Could you check a few things on this model? Use its own coordinates, in mm. Face numbers are marked on the shaded views. A direction names the side the tool comes from. Coordinates: 2 decimals unless noted, no trailing zeros. Order: outer loops, then holes, each group sorted by start corner. A loop starts at its lowest first (then second) coordinate and runs counter-clockwise, first axis right, second up. Notation, with made-up numbers: (-2, -22.5) - (3, -22.5) arc R16 cw to (3, 5.5) - close; hole circle Ø6 at (-19.5, 51.5). An arc over 180 degrees is marked (long way). Answer as a JSON object with one key per item and string values. Group by question number.
(1) Imagine slicing it at D-D, the plane y = 109.5. Write out the boundary of the cut face in (x, z), and give its area (3 significant figures).
(2) Imagine slicing it at A-A, the plane z = -72. Write out the boundary of the cut face in (x, y), and give its area (3 significant figures).
(3) Please list where these lines run through material, in increasing order: probe 1 along Y at (x, z) = (-10, -51); probe 2 along Z at (x, y) = (-9, 146); probe 3 along Y at (x, z) = (42, -43).
(4) Which directions (+Z, -Z, +X, -X, +Y, -Y) give clear straight access to the entire face, cutting with the end or side of a thin tool? Please do the marked faces 1, 2, 3 and 4.
(5) We'd pull the mould along Y, two halves only. Please class the marked faces 5, 6 and 7: pulls with the +Y half, pulls with the -Y half, needs draft (parallel to the pull), parting line crosses it, or undercut.
(6) Imagine slicing it at B-B, the plane y = -146. Write out the boundary of the cut face in (x, z).
(7) Imagine slicing it at C-C, the plane x = -34.5. Write out the boundary of the cut face in (y, z).
(8) Will these pins go through, and if not, where does the flat tip stop? P1, Ø25, axis at y = 106, z = -34, coming from the -X side; P2, Ø3, axis at x = 24, y = -40.5, coming from the -Z side; P3, Ø12, axis at x = 47, z = -115.5, coming from the -Y side; P4, Ø12, axis at x = -72.5, y = -69, coming from the +Z side.
from build123d import *

# Parameters (mm, degrees)
BOSS_EXTRUDE1_DEPTH                              = 140
SKETCH2_W                                        = 55
SKETCH2_H                                        = 50
BOSS_EXTRUDE2_DEPTH                              = 88
CUT_EXTRUDE1_DEPTH                               = 256.480429779
RIB1_REACH                                       = 244.701
SKETCH4_WALL_W                                   = 572.27930611
SKETCH4_WALL_H                                   = 12
SKETCH5_R                                        = 12.5
BOSS_EXTRUDE3_DEPTH                              = 70
CSK_FOR_M10_FLAT_HEAD_MACHINE_SCREW1_D           = 11
CSK_FOR_M10_FLAT_HEAD_MACHINE_SCREW1_CSINK_D     = 20
CSK_FOR_M10_FLAT_HEAD_MACHINE_SCREW1_CSINK_ANGLE = 90
F_10_0MM_DOWEL_HOLE2_D                           = 13.5
F_10_0MM_DOWEL_HOLE2_DEPTH                       = 35.944190822
F_10_0MM_DOWEL_HOLE2_TIP                         = 4.055809178
CBORE_FOR_M14_HEX_HEAD_BOLT1_D                   = 15.5
CBORE_FOR_M14_HEX_HEAD_BOLT1_CBORE_D             = 27.25
CBORE_FOR_M14_HEX_HEAD_BOLT1_CBORE_DEPTH         = 9.25
CUT_EXTRUDE2_START                               = -20
CUT_EXTRUDE2_DEPTH                               = 20


with BuildPart() as part:
    # Sketch1 → Boss-Extrude1 (new body)
    with BuildSketch(Plane.XY):
        with BuildLine():
            Line((0, 40), (-93.829632846, 40))
            ThreePointArc((-93.829632846, 40), (-80.04994488, 63.213972543), (-60.663003552, 82))
            Line((-60.663003552, 82), (60.663003552, 82))
            ThreePointArc((60.663003552, 82), (63.213972543, -80.04994488), (-93.829632846, -40))
            Line((-93.829632846, -40), (0, -40))
            ThreePointArc((0, -40), (40, 0), (0, 40))
        make_face()
    extrude(amount=-BOSS_EXTRUDE1_DEPTH)

    # Sketch2 → Boss-Extrude2 (add)
    with BuildSketch(Plane(origin=(0, 170, 0), x_dir=(1, 0, 0), z_dir=(0, 1, 0))):
        with Locations((0, 35)):
            Rectangle(SKETCH2_W, SKETCH2_H)
    extrude(amount=-BOSS_EXTRUDE2_DEPTH)

    # Sketch3 → Cut-Extrude1 (cut, through all)
    with BuildSketch(Plane.ZY.offset(27.5)):
        with BuildLine():
            ThreePointArc((-60, 145), (-52.67766953, 162.67766953), (-35, 170))
            Line((-35, 170), (-60, 170))
            Line((-60, 170), (-60, 145))
        make_face()
        with BuildLine():
            ThreePointArc((-35, 170), (-17.32233047, 162.67766953), (-10, 145))
            Line((-10, 145), (-10, 170))
            Line((-10, 170), (-35, 170))
        make_face()
    extrude(amount=-CUT_EXTRUDE1_DEPTH, mode=Mode.SUBTRACT)

    # Sketch4 wall → Rib1 (add, up to next)
    with BuildSketch(Plane(origin=(0, 106, -95), x_dir=(0, -0.565528355552, -0.824728851846), z_dir=(0, 0.824728851846, -0.565528355552)), mode=Mode.PRIVATE) as rib1_sk1:
        Rectangle(SKETCH4_WALL_W, SKETCH4_WALL_H)
    rib1_tool1 = extrude(rib1_sk1.sketch, amount=-RIB1_REACH, mode=Mode.PRIVATE) - part.part
    add(rib1_tool1.solids().sort_by_distance((0, 106, -95))[0])

    # Sketch5 → Boss-Extrude3 (add)
    with BuildSketch(Plane.XY.offset(-10)):
        with BuildLine():
            Line((-27.5, -98.222960656), (-27.5, -119.775011916))
            ThreePointArc((-27.5, -119.775011916), (-21.697882646, -177.19618388), (34.154451435, -162.657534247))
            Line((34.154451435, -162.657534247), (91.677738062, -44.712328767))
            ThreePointArc((91.677738062, -44.712328767), (41.779689407, -93.050833167), (-27.5, -98.222960656))
        make_face()
        with Locations((0, -146)):
            Circle(SKETCH5_R, mode=Mode.SUBTRACT)
    extrude(amount=-BOSS_EXTRUDE3_DEPTH)

    # CSK for M10 Flat Head Machine Screw1 (through all)
    with Locations(Plane.XY):
        with Locations((37.094348496, -59.363366731), (37.094348496, 59.363366731)):
            CounterSinkHole(CSK_FOR_M10_FLAT_HEAD_MACHINE_SCREW1_D / 2, CSK_FOR_M10_FLAT_HEAD_MACHINE_SCREW1_CSINK_D / 2, counter_sink_angle=CSK_FOR_M10_FLAT_HEAD_MACHINE_SCREW1_CSINK_ANGLE)

    # Ø10.0mm Dowel Hole2
    with Locations(Plane.XY):
        with Locations((-20, 59.363366731), (-20, -59.363366731)):
            Hole(F_10_0MM_DOWEL_HOLE2_D / 2, depth=F_10_0MM_DOWEL_HOLE2_DEPTH)
            with Locations((0, 0, -(F_10_0MM_DOWEL_HOLE2_DEPTH + F_10_0MM_DOWEL_HOLE2_TIP / 2))):  # 118° drill point
                Cone(0, F_10_0MM_DOWEL_HOLE2_D / 2, F_10_0MM_DOWEL_HOLE2_TIP, mode=Mode.SUBTRACT)

    # CBORE for M14 Hex Head Bolt1 (through all)
    with Locations(Plane(origin=(27.5, 0, 0), x_dir=(0, 0, -1), z_dir=(1, 0, 0))):
        with Locations((35, 145)):
            CounterBoreHole(CBORE_FOR_M14_HEX_HEAD_BOLT1_D / 2, CBORE_FOR_M14_HEX_HEAD_BOLT1_CBORE_D / 2, CBORE_FOR_M14_HEX_HEAD_BOLT1_CBORE_DEPTH)

    # Sketch14 → Cut-Extrude2 (cut)
    with BuildSketch(Plane(origin=(0, 0, -140), x_dir=(-1, 0, 0), z_dir=(0, 0, -1)).offset(CUT_EXTRUDE2_START)):
        with BuildLine():
            Line((0, 50), (88.904443084, 50))
            ThreePointArc((88.904443084, 50), (102, 0), (88.904443084, -50))
            Line((88.904443084, -50), (0, -50))
            ThreePointArc((0, -50), (-50, 0), (0, 50))
        make_face()
    extrude(amount=CUT_EXTRUDE2_DEPTH, mode=Mode.SUBTRACT)


solid = part.part
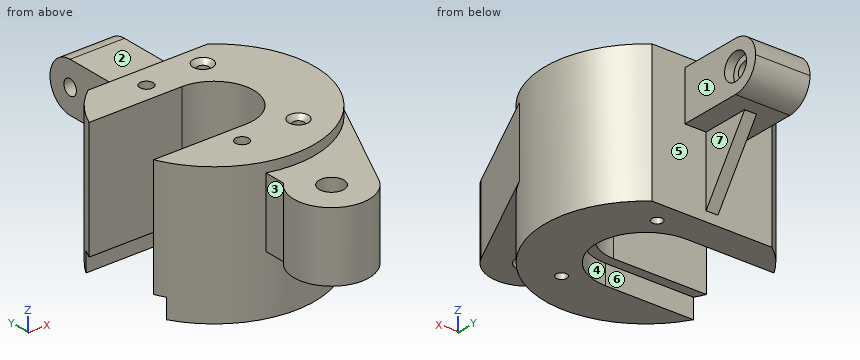
Result set:
{
 "1": {"outline": "(-27.5, -60) - (-6, -60) - (-6, -89.9) - (6, -89.9) - (6, -60) - (27.5, -60) - (27.5, -10) - (-27.5, -10) - close", "area": "3,110 mm^2"},
 "2": {"outline": "(-93.83, -40) arc R102 ccw to (-27.5, -98.22) - (-27.5, -119.78) arc R38 ccw (long way) to (34.15, -162.66) - (91.68, -44.71) arc R102 ccw to (60.66, 82) - (6, 82) - (6, 121.77) - (-6, 121.77) - (-6, 82) - (-60.66, 82) arc R102 ccw to (-93.83, 40) - (0, 40) arc R40 cw to (0, -40) - close; hole circle Ø25 at (0, -146); hole circle Ø11 at (37.09, -59.36); hole circle Ø11 at (37.09, 59.36)", "area": "27,100 mm^2"},
 "3": {"probe 1": "y = -182.66 to -153.5, -138.5 to -40, 40 to 164.21", "probe 2": "z = -59.98 to -42.69, -27.31 to -10.02", "probe 3": "y = -146.57 to -61.85, -56.88 to 56.88, 61.85 to 82"},
 "4": {"face 1": "+Z, -Z, +X, +Y", "face 2": "+Z, +X, -X, +Y", "face 3": "+Z, -Z, -X", "face 4": "-Z, -X"},
 "5": {"face 5": "pulls with the +Y half", "face 6": "undercut", "face 7": "needs draft"},
 "6": {"outline": "(-38, -80) - (-12.5, -80) - (-12.5, -10) - (-38, -10) - close; (12.5, -80) - (42.28, -80) - (42.28, -10) - (12.5, -10) - close"},
 "7": {"outline": "(-161.93, -80) - (-130.07, -80) - (-130.07, -10) - (-161.93, -10) - close; (-95.99, -140) - (-50, -140) - (-50, -120) - (-40, -120) - (-40, 0) - (-95.99, 0) - close; (40, -120) - (50, -120) - (50, -140) - (82, -140) - (82, 0) - (40, 0) - close"},
 "8": {"P1": "stops at x = -27.5", "P2": "stops at z = -120", "P3": "stops at y = -93.4", "P4": "stops at z = 0"}
}
